Autodesk Inventor part; units mm, degrees
ref_plane "YZ Plane" through (0, 0, 0) normal (1, 0, 0) x (0, 1, 0)
ref_plane "XZ Plane" through (0, 0, 0) normal (0, 1, 0) x (-1, 0, 0)
ref_plane "XY Plane" through (0, 0, 0) normal (0, 0, 1) x (1, 0, 0)
sketch "Sketch1" plane through (0, 0, 0) normal (0, 1, 0) x (-1, 0, 0)
  line L0 (-25, 25) -> (25, 25)
  line L1 (25, 25) -> (25, -25)
  line L2 (25, -25) -> (-25, -25)
  line L3 (-25, -25) -> (-25, 25)
  line L4 (-25, 25) -> (25, -25) construction
  line L5 (25, 25) -> (-25, -25) construction
  line L6 (-17.4, 17.4) -> (17.4, 17.4)
  line L7 (17.4, 17.4) -> (17.4, -17.4)
  line L8 (17.4, -17.4) -> (-17.4, -17.4)
  line L9 (-17.4, -17.4) -> (-17.4, 17.4)
  line L10 (-17.4, 17.4) -> (17.4, -17.4) construction
  line L11 (17.4, 17.4) -> (-17.4, -17.4) construction
  point P0 (0, 0)
  dimension "d0" = 50
  dimension "d1" = 50
  dimension "d2" = 34.8
  dimension "d3" = 34.8
extrude "Extrusion1" add sketch "Sketch1" along normal blind 5
extrude "Extrusion2" add sketch "Sketch1" along normal blind 15 contours L6 L7 L8 L9
sketch "Sketch3" plane through (0, 15, 0) normal (0, 1, 0) x (1, 0, 0)
  point P0 (0, 0)
ref_plane "Work Plane6" through (0, 5, 17.4) normal (-1, 0, 0) x (0, 0, 1)
ref_plane "Work Plane7" through (-17.4, 5, 0) normal (0, 0, 1) x (1, 0, 0)
sketch "Sketch6" plane through (0, 0, 0) normal (0, -1, 0) x (1, 0, 0)
  line L0 (-25, 25) -> (25, 25)
  line L1 (-5, -25) -> (5, -25)
  line L2 (5, -25) -> (5, 25)
  line L3 (5, 25) -> (-5, 25)
  line L4 (-5, 25) -> (-5, -25)
  line L5 (-5, -25) -> (5, 25) construction
  line L6 (5, -25) -> (-5, 25) construction
  line L7 (25, 25) -> (25, -25)
  line L8 (-25, -5) -> (25, -5)
  line L9 (25, -5) -> (25, 5)
  line L10 (25, 5) -> (-25, 5)
  line L11 (-25, 5) -> (-25, -5)
  line L12 (-25, -5) -> (25, 5) construction
  line L13 (25, -5) -> (-25, 5) construction
  point P0 (0, 0)
  point P1 (-5, -5)
  point P2 (5, -5)
  point P3 (5, 5)
  point P4 (-5, 5)
  dimension "d14" = 10
extrude "Extrusion5" add sketch "Sketch6" along normal blind 2 contours L0 L2 L10 L4 | L10 L2 L8 L4 | L4 L8 L11 L10 | L10 L7 L8 L2 | L8 L2 L1 L4
sketch "Sketch7" plane through (-25, 0, 25) normal (-1, 0, 0) x (0, 0, 1)
  line L0 (-20, -2) -> (-30, -2)
  line L1 (-7.6, 5) -> (-42.4, 5)
  line L2 (-20, -2) -> (-30, -2)
  line L3 (-30, -2) -> (-30, 5)
  line L4 (-30, 5) -> (-20, 5)
  line L5 (-20, 5) -> (-20, -2)
  point P0 (-25, 0)
  dimension "d17" = 10
extrude "Extrusion6" add sketch "Sketch7" along normal blind 2
mirror "Mirror4" about plane through (0, 5, 17.4) normal (-1, 0, 0) of "Extrusion6"
sketch "Sketch8" plane through (25, 5, -25) normal (0, 0, -1) x (-1, 0, 0)
  line L0 (30, -7) -> (20, -7)
  line L1 (0, 0) -> (50, 0)
  line L2 (20, -7) -> (30, -7)
  line L3 (30, -7) -> (30, 0)
  line L4 (30, 0) -> (20, 0)
  line L5 (20, 0) -> (20, -7)
  point P0 (25, -5)
  dimension "d20" = 10
extrude "Extrusion7" add sketch "Sketch8" along normal blind 2
mirror "Mirror5" about plane through (-17.4, 5, 0) normal (0, 0, 1) of "Extrusion7"
sketch "Sketch9" plane through (0, 0, 0) normal (0, -1, 0) x (1, 0, 0)
  line L0 (-27, 27) -> (27, 27)
  line L1 (27, 27) -> (27, -27)
  line L2 (27, -27) -> (-27, -27)
  line L3 (-27, -27) -> (-27, 27)
  line L4 (-27, 27) -> (27, -27) construction
  line L5 (27, 27) -> (-27, -27) construction
  point P0 (0, 0)
  dimension "d24" = 54
  dimension "d25" = 54
extrude "Extrusion8" cut sketch "Sketch9" along normal blind 6.75
sketch "Sketch10" plane through (0, 15, 0) normal (0, 1, 0) x (1, 0, 0)
  line L0 (12.5, -12.5) -> (-12.5, -12.5)
  line L1 (-12.5, -12.5) -> (-12.5, 12.5)
  line L2 (-12.5, 12.5) -> (12.5, 12.5)
  line L3 (12.5, 12.5) -> (12.5, -12.5)
  line L4 (12.5, -12.5) -> (-12.5, 12.5) construction
  line L5 (-12.5, -12.5) -> (12.5, 12.5) construction
  point P0 (0, 0)
  dimension "d28" = 25
  dimension "d29" = 25
extrude "Extrusion9" cut sketch "Sketch10" against normal blind 11.45
sketch "Sketch11" plane through (-17.4, 5, 17.4) normal (-1, 0, 0) x (0, 0, 1)
  line L0 (-17.5, 0.0162) -> (-17.5, 3.5)
  circle A0 centre (-17.5, 3.5) radius 1.75
  line L1 (0, 0) -> (-34.8, 0)
  line L2 (-17.4, 0) -> (-18.8366, 0)
  point P0 (-17.4, -5)
  dimension "d34" = 3.5
  dimension "d57" = 3.5
extrude "Extrusion10" cut sketch "Sketch11" against normal through all
sketch "Sketch14" plane through (27, 0, -5) normal (1, 0, 0) x (0, 0, -1)
  line L0 (12.4, 5) -> (-22.4, 5)
  line L1 (-15, 0) -> (5, 0)
  line L2 (5, 0) -> (5, 5)
  line L3 (5, 5) -> (-15, 5)
  line L4 (-15, 5) -> (-15, 0)
  line L5 (-15, 0) -> (5, 5) construction
  line L6 (5, 0) -> (-15, 5) construction
  point P0 (-5, 0)
  point P1 (-5, 2.5)
  dimension "d43" = 20
extrude "Extrusion13" cut sketch "Sketch14" against normal blind 2
pattern_circular "Circular Pattern1" count 4 over 360 about axis through (0, -10, 0) along (0, 1, 0) of "Extrusion13"
sketch "Sketch15" plane through (17.4, 5, -17.4) normal (0, 0, -1) x (-1, 0, 0)
  line L0 (42.4, 0) -> (-7.6, 0)
  line L1 (17.4, 0) -> (17.4, 3.5)
  circle A0 centre (17.4, 3.5) radius 1.75
  point P0 (17.4, -5)
  point P1 (27.4, 0)
  point P2 (7.4, 0)
  dimension "d49" = 3.5
  dimension "d50" = 3.5
extrude "Extrusion14" cut sketch "Sketch15" against normal through all
chamfer "Chamfer1" distance 4 distance2 4 4 edges at (0, 15, -17.4) (-17.4, 15, 0) (0, 15, 17.4) (17.4, 15, 0) measured on face at (15.7667, 15, 4.1667)
fillet "Fillet1" radius 2 4 edges at (0, 11, -17.4) (-17.4, 11, 0) (0, 11, 17.4) (17.4, 11, 0)
properties part number "Pokrywka"
Geometry check sheet. Reference: the model listing, model coordinates, mm. A direction names the side the tool comes from. Coordinates: 2 decimals unless noted, no trailing zeros. Order: outer loops, then holes, each group sorted by start corner. A loop starts at its lowest first (then second) coordinate and runs counter-clockwise, first axis right, second up. Notation, with made-up numbers: (9, -23) - (24, -23) arc R20 cw to (24, 10) - close; hole circle Ø1 at (63.5, 51.5). An arc over 180 degrees is marked (long way). Answer as a JSON object with one key per item and string values. Group by question number.
Item 1: Sectioned sample at B-B, the plane x = 10. Record the cut outline in (y, z), and give its area (3 significant figures).
Item 2: Scan lines: probe 1 along X at (y, z) = (8.5, -15.9); probe 2 along Z at (x, y) = (15.8, 8.5); probe 3 along Z at (x, y) = (-11.5, 9). Record each from-to range of solid material in increasing order.
Item 3: Sectioned sample at C-C, the plane y = 5.75. Record the cut outline in (x, z).
Item 4: Sectioned sample at A-A, the plane y = 8.5. Record the cut outline in (x, z).
Item 5: Sectioned sample at D-D, the plane z = -8.5. Record the cut outline in (x, y).
Item 6: Tool access check on faces 1 (the face through (17.4, 6, 0)), 2 (the face through (0, 6, -17.4)), 3 (the face through (12.5, 11, 0)), 4 (the face through (0, 6, 17.4)). Record the directions out of +Z, -Z, +X, -X, +Y, -Y that give a thin tool (end or side, any length) a straight path to the whole face; none if there is none.
Item 7: Draft check along Z on faces 5 (the face through (9.08, 10.93, -17.25)), 6 (the face through (-17.25, 10.93, -9.13)), 7 (the face through (0, 11, 12.5)). Enter one of: +Z half, -Z half, draft (parallel to the pull), parting line (faces both ways), or undercut.
Item 8: Depth check by flat-ended pin: pin 1 Ø1 at (x, z) = (14, 2) entering from +Y; pin 2 Ø1.6 at (x, y) = (3.5, 8) entering from +Z; pin 3 Ø12.5 at (x, z) = (1, 3.5) entering from +Y; pin 4 Ø3 at (x, y) = (0, 8.5) entering from -Z. Enter the tip coordinate at first touch or a pass-through.
Resolved:
{
 "1": {"outline": "(0, -25) - (5, -25) - (5, -17.4) - (10.17, -17.4) arc R2 ccw to (11.59, -16.81) - (15, -13.4) - (15, -12.5) - (3.55, -12.5) - (3.55, 12.5) - (15, 12.5) - (15, 13.4) - (11.59, 16.81) arc R2 ccw to (10.17, 17.4) - (5, 17.4) - (5, 25) - (0, 25) - close", "area": "296 mm^2"},
 "2": {"probe 1": "-17.4 to -1.75, 1.75 to 17.4", "probe 2": "-17.4 to -1.85, 1.65 to 17.4", "probe 3": "-17.4 to -12.5, 12.5 to 17.4"},
 "3": {"outline": "(-17.4, -17.4) - (17.4, -17.4) - (17.4, 17.4) - (-17.4, 17.4) - close; hole (-12.5, -12.5) - (12.5, -12.5) - (12.5, 12.5) - (-12.5, 12.5) - close"},
 "4": {"outline": "(-17.4, -17.4) - (-1.75, -17.4) - (-1.75, -12.5) - (-12.5, -12.5) - (-12.5, -1.85) - (-17.4, -1.85) - close; (-17.4, 1.65) - (-12.5, 1.65) - (-12.5, 12.5) - (-1.75, 12.5) - (-1.75, 17.4) - (-17.4, 17.4) - close; (1.75, -17.4) - (17.4, -17.4) - (17.4, -1.85) - (12.5, -1.85) - (12.5, -12.5) - (1.75, -12.5) - close; (1.75, 12.5) - (12.5, 12.5) - (12.5, 1.65) - (17.4, 1.65) - (17.4, 17.4) - (1.75, 17.4) - close"},
 "5": {"outline": "(-25, 0) - (25, 0) - (25, 5) - (17.4, 5) - (17.4, 10.17) arc R2 ccw to (16.81, 11.59) - (13.4, 15) - (12.5, 15) - (12.5, 3.55) - (-12.5, 3.55) - (-12.5, 15) - (-13.4, 15) - (-16.81, 11.59) arc R2 ccw to (-17.4, 10.17) - (-17.4, 5) - (-25, 5) - close"},
 "6": {"face 1": "+Z, -Z, +X, +Y", "face 2": "-Z, +X, -X, +Y", "face 3": "+Y", "face 4": "+Z, +X, -X, +Y"},
 "7": {"face 5": "-Z half", "face 6": "draft", "face 7": "undercut"},
 "8": {"pin 1": "y = 14.9", "pin 2": "z = 17.4", "pin 3": "y = 3.55", "pin 4": "through"}
}
